Geometry: see drawing. Coordinates: mm, zero at the bounding-box minimum. A direction names the side the tool comes from. Coordinates: 2 decimals unless noted, no trailing zeros. Loops run counter-clockwise (first coordinate to the right, second up) from the corner with the lowest first, then second, coordinate; pieces in that order, holes last. Notation, with made-up numbers: (33, 28) - (55, 28) arc R22 ccw to (55, 62) - close; hole circle Ø7 at (54, -7.5). An arc over 180 degrees is marked (long way). Answer in a Markdown table with one row per item.
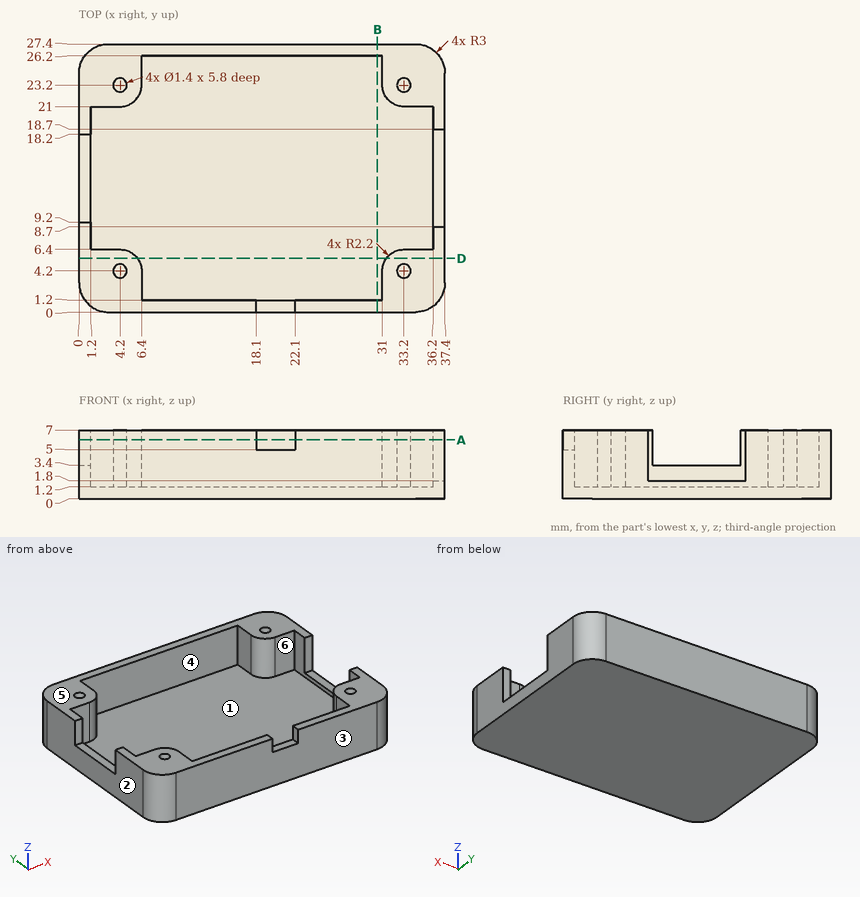
(1) Pull-direction query (Y, two-part tool) for the marked faces 1, 2, 3 and 4; classes: pulls with the +Y half, pulls with the -Y half, needs draft (parallel to the pull), parting line crosses it, or undercut.
Verdict:
| item | result |
|---|---|
| face 1 | undercut |
| face 2 | needs draft |
| face 3 | pulls with the -Y half |
| face 4 | undercut |
(2) First-contact query: pin 1 Ø1 at (y, z) = (0.5, 6) entering from +X; pin 2 Ø1.3 at (x, y) = (36.5, 15.5) entering from +Z; pin 3 Ø1 at (x, y) = (0.5, 13.5) entering from +Z. Flat tips, straight axial feed; report the tip coordinate or a pass-through.
Verdict:
| item | result |
|---|---|
| pin 1 | stops at x = 36.64 |
| pin 2 | stops at z = 1.8 |
| pin 3 | stops at z = 3.4 |
(3) Cut plane D-D on y = 5.5. Output: boundary loops of the cut face in (x, z).
Verdict:
| item | result |
|---|---|
| outline | (0, 0) - (37.4, 0) - (37.4, 7) - (31.43, 7) - (31.43, 1.2) - (5.97, 1.2) - (5.97, 7) - (0, 7) - close |
(4) Cut plane A-A on z = 6. State how many separate pieces and enclosed holes the cut face has, then the cut area to 3 significant figures.
Verdict:
| item | result |
|---|---|
| separate pieces | 3 |
| enclosed holes | 4 |
| area | 212 mm² |
(5) Ray query, probe 1 along Y at (x, z) = (33.2, 3.8); probe 2 along Y at (x, z) = (25.5, 5.5); probe 3 along X at (y, z) = (4, 1.5). Return the intervals inside material, ascending.
Verdict:
| item | result |
|---|---|
| probe 1 | y = 0 to 3.5, 4.9 to 6.4, 21 to 22.5, 23.9 to 27.4 |
| probe 2 | y = 0 to 1.2, 26.2 to 27.4 |
| probe 3 | x = 0 to 3.53, 4.87 to 6.4, 31 to 32.53, 33.87 to 37.4 |
(6) Cut plane B-B on x = 30.5. Output: boundary loops of the cut face in (y, z), then the cut area to 3 significant figures.
Verdict:
| item | result |
|---|---|
| outline | (0, 0) - (27.4, 0) - (27.4, 7) - (26.2, 7) - (26.2, 1.2) - (1.2, 1.2) - (1.2, 7) - (0, 7) - close |
| area | 46.8 mm² |
(7) Access query for the marked faces 5 and 6. Directions: +Z, -Z, +X, -X, +Y, -Y. A direction counts if a zero-diameter tool reaches every point of the face in a straight line with its end or side. Return the directions, or none.
Verdict:
| item | result |
|---|---|
| face 5 | +Z, +X, -X, +Y, -Y |
| face 6 | +Z |
